CAD build for the part. Positions are in the model's coordinates, mm. A direction names the side the tool comes from. Coordinates: 2 decimals unless noted, no trailing zeros. Write each loop counter-clockwise with the first axis right and the second up, starting at its lowest first coordinate (ties: lowest second). Pieces come first, ordered by that corner, then holes. Notation, with made-up numbers: (2.5, 83.25) -> (31.5, 83.25) arc R26 ccw to (31.5, 115.25) -> close; hole circle Ø6 at (-19.5, 37). An arc over 180 degrees is marked (long way). Answer as CSV lines item,"result".
```python
from build123d import *

# Parameters (mm, degrees)
SKETCH1_W           = 50
SKETCH1_H           = 40
BOSS_EXTRUDE1_DEPTH = 3
SKETCH6_R           = 2
CUT_EXTRUDE9_DEPTH  = 5
SKETCH16_W          = 14.8
SKETCH16_H          = 3
CUT_EXTRUDE10_DEPTH = 0.5
SKETCH21_R          = 14.25
CUT_EXTRUDE15_DEPTH = 4
CUT_EXTRUDE16_START = -4
CUT_EXTRUDE16_DEPTH = 4
SKETCH33_W          = 4
SKETCH33_H          = 35
CUT_EXTRUDE23_DEPTH = 5
SKETCH34_W          = 49.986920535
SKETCH34_H          = 3
BOSS_EXTRUDE2_DEPTH = 3
SKETCH35_W          = 50
SKETCH35_H          = 3
BOSS_EXTRUDE3_DEPTH = 3
SKETCH36_W          = 46
SKETCH36_H          = 3
BOSS_EXTRUDE4_DEPTH = 4
SKETCH38_W          = 3
SKETCH38_H          = 46
BOSS_EXTRUDE5_DEPTH = 25
SKETCH39_W          = 45.535565308
SKETCH39_H          = 3
BOSS_EXTRUDE6_DEPTH = 15
SKETCH40_W          = 46
SKETCH40_H          = 3
BOSS_EXTRUDE7_DEPTH = 15
SKETCH41_W          = 0.464434692
SKETCH41_H          = 3
BOSS_EXTRUDE8_DEPTH = 15
SKETCH42_R          = 2
CUT_EXTRUDE24_DEPTH = 15
SKETCH43_R          = 2
CUT_EXTRUDE25_DEPTH = 15


with BuildPart() as part:
    # Sketch1 → Boss-Extrude1 (new body)
    with BuildSketch(Plane(origin=(0, 0, 0), x_dir=(1, 0, 0), z_dir=(0, 1, 0))):
        with Locations((1.920937393, -5.615172506)):
            Rectangle(SKETCH1_W, SKETCH1_H)
    extrude(amount=BOSS_EXTRUDE1_DEPTH)

    # Sketch6 → Cut-Extrude9 (cut)
    with BuildSketch(Plane.XZ):
        with Locations(Location((6.920937393, 23.115172506, 0), (0, 0, 270))):
            Circle(SKETCH6_R)
        with Locations(Location((6.920937393, -11.884827494, 0), (0, 0, 270))):
            Circle(SKETCH6_R)
        with BuildLine():
            Line((24.420937393, 13.015172506), (18.923020545, 13.015172506))
            ThreePointArc((18.923020545, 13.015172506), (-7.179062607, 5.615172506), (18.923020545, -1.784827494))
            Line((18.923020545, -1.784827494), (24.420937393, -1.784827494))
            Line((24.420937393, -1.784827494), (24.420937393, 5.615172506))
            Line((24.420937393, 5.615172506), (24.420937393, 13.015172506))
        make_face()
    extrude(amount=-CUT_EXTRUDE9_DEPTH, mode=Mode.SUBTRACT)

    # Sketch16 → Cut-Extrude10 (cut)
    with BuildSketch(Plane.ZY.offset(-24.420937393)):
        with Locations((5.615172506, 1.5)):
            Rectangle(SKETCH16_W, SKETCH16_H)
    extrude(amount=-CUT_EXTRUDE10_DEPTH, mode=Mode.SUBTRACT)

    # Sketch21 → Cut-Extrude15 (cut)
    with BuildSketch(Plane(origin=(0, 0, 0), x_dir=(-1, 0, 0), z_dir=(0, -1, 0))):
        with Locations((-6.920937393, -5.615172506)):
            Circle(SKETCH21_R)
    extrude(amount=-CUT_EXTRUDE15_DEPTH, mode=Mode.SUBTRACT)

    # Sketch22 → Cut-Extrude16 (cut)
    with BuildSketch(Plane(origin=(0, 3, 0), x_dir=(1, 0, 0), z_dir=(0, 1, 0)).offset(CUT_EXTRUDE16_START)):
        with BuildLine():
            ThreePointArc((21.106680727, 1.784827494), (20.39103932, 3.019158274), (19.568281538, 4.184827494))
            Line((19.568281538, 4.184827494), (17.266105347, 4.184827494))
            ThreePointArc((17.266105347, 4.184827494), (18.246250908, 3.03351374), (19.09888878, 1.784827494))
            Line((19.09888878, 1.784827494), (21.106680727, 1.784827494))
        make_face()
        with BuildLine():
            Line((17.266105347, -15.415172506), (19.568281538, -15.415172506))
            ThreePointArc((19.568281538, -15.415172506), (20.39103932, -14.249503286), (21.106680727, -13.015172506))
            Line((21.106680727, -13.015172506), (19.09888878, -13.015172506))
            ThreePointArc((19.09888878, -13.015172506), (18.246250908, -14.263858752), (17.266105347, -15.415172506))
        make_face()
    extrude(amount=CUT_EXTRUDE16_DEPTH, mode=Mode.SUBTRACT)

    # Sketch33 → Cut-Extrude23 (cut)
    with BuildSketch(Plane(origin=(0, 3, 0), x_dir=(1, 0, 0), z_dir=(0, 1, 0))):
        with Locations((6.920937393, -5.615172506)):
            Rectangle(SKETCH33_W, SKETCH33_H)
    extrude(amount=-CUT_EXTRUDE23_DEPTH, mode=Mode.SUBTRACT)

    # Sketch34 → Boss-Extrude2 (add)
    with BuildSketch(Plane(origin=(0, 0, -14.384827494), x_dir=(-1, 0, 0), z_dir=(0, 0, -1))):
        with Locations((-1.927477126, 1.5)):
            Rectangle(SKETCH34_W, SKETCH34_H)
    extrude(amount=BOSS_EXTRUDE2_DEPTH)

    # Sketch35 → Boss-Extrude3 (add)
    with BuildSketch(Plane.XY.offset(25.615172506)):
        with Locations((1.920937393, 1.5)):
            Rectangle(SKETCH35_W, SKETCH35_H)
    extrude(amount=BOSS_EXTRUDE3_DEPTH)

    # Sketch36 → Boss-Extrude4 (add)
    with BuildSketch(Plane(origin=(26.920937393, 0, 0), x_dir=(0, 0, -1), z_dir=(1, 0, 0))):
        with Locations((-5.615172506, 1.5)):
            Rectangle(SKETCH36_W, SKETCH36_H)
    extrude(amount=BOSS_EXTRUDE4_DEPTH)

    # Sketch38 → Boss-Extrude5 (add)
    with BuildSketch(Plane(origin=(0, 3, 0), x_dir=(1, 0, 0), z_dir=(0, 1, 0))):
        with Locations((29.420937393, -5.615172506)):
            Rectangle(SKETCH38_W, SKETCH38_H)
        with Locations((-21.565983142, -5.615172506)):
            Rectangle(SKETCH38_W, SKETCH38_H)
    extrude(amount=BOSS_EXTRUDE5_DEPTH)

    # Sketch39 → Boss-Extrude6 (add)
    with BuildSketch(Plane.ZY.offset(23.065983142)):
        with Locations((5.38295516, 26.5)):
            Rectangle(SKETCH39_W, SKETCH39_H)
    extrude(amount=BOSS_EXTRUDE6_DEPTH)

    # Sketch40 → Boss-Extrude7 (add)
    with BuildSketch(Plane(origin=(30.920937393, 0, 0), x_dir=(0, 0, -1), z_dir=(1, 0, 0))):
        with Locations((-5.615172506, 26.5)):
            Rectangle(SKETCH40_W, SKETCH40_H)
    extrude(amount=BOSS_EXTRUDE7_DEPTH)

    # Sketch41 → Boss-Extrude8 (add)
    with BuildSketch(Plane.ZY.offset(23.065983142)):
        with Locations((28.38295516, 26.5)):
            Rectangle(SKETCH41_W, SKETCH41_H)
    extrude(amount=BOSS_EXTRUDE8_DEPTH)

    # Sketch42 → Cut-Extrude24 (cut)
    with BuildSketch(Plane.XZ.offset(-25)):
        with Locations(Location((38.420937393, 20.419520332, 0), (0, 0, 270))):
            Circle(SKETCH42_R)
        with Locations(Location((38.420937393, -8.692413747, 0), (0, 0, 270))):
            Circle(SKETCH42_R)
    extrude(amount=-CUT_EXTRUDE24_DEPTH, mode=Mode.SUBTRACT)

    # Sketch43 → Cut-Extrude25 (cut)
    with BuildSketch(Plane.XZ.offset(-25)):
        with Locations(Location((-30.565983142, 20.419520332, 0), (0, 0, 270))):
            Circle(SKETCH43_R)
        with Locations(Location((-30.565983142, -8.692413747, 0), (0, 0, 270))):
            Circle(SKETCH43_R)
    extrude(amount=-CUT_EXTRUDE25_DEPTH, mode=Mode.SUBTRACT)


solid = part.part
```
Item 1: 3-axis set-ups, long thin cutter, end or side, ignore diameter. For faces 1 (the flat face through (45.921, 27, 6)), 2 (the flat face through (23, 1, 13.015)), 3 (the flat face through (38, 25, 6)): which of +Z, -Z, +X, -X, +Y, -Y reach the whole face in a straight line?
Answer below:
face 1,"+Z, -Z, +X, +Y, -Y"
face 2,"+Y, -Y"
face 3,"+Z, -Z, +X, -Y"
Item 2: Saw through at D-D on y = 26. Give the cut face in (x, z).
Answer below:
outline,"(-38.07, -17.38) -> (-20.07, -17.38) -> (-20.07, 28.62) -> (-38.07, 28.62) -> close; (27.92, -17.38) -> (45.92, -17.38) -> (45.92, 28.62) -> (27.92, 28.62) -> close; hole circle Ø4 at (-30.57, -8.69); hole circle Ø4 at (-30.57, 20.42); hole circle Ø4 at (38.42, -8.69); hole circle Ø4 at (38.42, 20.42)"
Item 3: Two-plate mould, pull along Z, no slides. Class faces 4 (the flat face through (8.921, 2, -10)), 5 (the flat face through (1, 2.5, 28.615)), 6 (the flat face through (-7, 3, 1)), 7 (the flat face through (6.8, 2.5, -17.385)): pulls with the +Z half, pulls with the -Z half, needs draft (parallel to the pull), parting line crosses it, or undercut.
Answer below:
face 4,"undercut"
face 5,"pulls with the +Z half"
face 6,"needs draft"
face 7,"pulls with the -Z half"
Item 4: Saw through at A-A on y = 8.25. Give the cut face in (x, z).
Answer below:
outline,"(-23.07, -17.38) -> (-20.07, -17.38) -> (-20.07, 28.62) -> (-23.07, 28.62) -> close; (27.92, -17.38) -> (30.92, -17.38) -> (30.92, 28.62) -> (27.92, 28.62) -> close"
Item 5: Saw through at B-B on x = 24. Give the cut face in (y, z), and give its area (3 significant figures).
Answer below:
outline,"(0, -17.38) -> (3, -17.38) -> (3, -1.78) -> (0, -1.78) -> close; (0, 13.02) -> (3, 13.02) -> (3, 28.62) -> (0, 28.62) -> close"
area,"93.6 mm2"
Item 6: Wall check: line 1 (X direction, y = 7.25, z = -4); line 2 (Y direction, x = -15, z = 25); line 3 (X direction, y = 26, z = -11.5). Give the ranges that are in metal, low to high. Write a range as from..to.
Answer below:
line 1,"x = -23.07..-20.07, 27.92..30.92"
line 2,"y = 0..3"
line 3,"x = -38.07..-20.07, 27.92..45.92"
Item 7: Flat gauge pins, fed straight in: pin 1 (4.5 mm diameter, centred on x = -30, z = 7, fed in from -Y); pin 2 (2.5 mm diameter, centred on y = 2, z = 6.5, fed in from -X); pin 3 (3.5 mm diameter, centred on x = 38.42, z = -8.69, fed in from +Y); pin 4 (12.5 mm diameter, centred on y = 9.5, z = -2, fed in from +X). Where does each tip first touch, or does it go through?
Answer below:
pin 1,"stops at y = 25"
pin 2,"stops at x = -23.08"
pin 3,"passes through"
pin 4,"stops at x = 30.92"
